Autodesk Inventor part; units mm, degrees
ref_plane "YZ Plane" through (0, 0, 0) normal (1, 0, 0) x (0, 1, 0)
ref_plane "XZ Plane" through (0, 0, 0) normal (0, 1, 0) x (-1, 0, 0)
ref_plane "XY Plane" through (0, 0, 0) normal (0, 0, 1) x (1, 0, 0)
sketch "Sketch1" plane through (0, 0, 0) normal (0, 0, 1) x (1, 0, 0)
  line L0 (0, 0) -> (50.8, 0)
  line L1 (50.8, 0) -> (50.8, 25.4)
  line L2 (50.8, 25.4) -> (0, 25.4)
  line L3 (0, 25.4) -> (0, 0)
  line L4 (3.175, 3.175) -> (47.625, 3.175)
  line L5 (47.625, 3.175) -> (47.625, 22.225)
  line L6 (47.625, 22.225) -> (3.175, 22.225)
  line L7 (3.175, 22.225) -> (3.175, 3.175)
  dimension "d0" = 50.8
  dimension "d1" = 25.4
  dimension "d2" = 3.175
  dimension "d3" = 3.175
  dimension "d4" = 3.175
  dimension "d5" = 3.175
extrude "Extrusion1" add sketch "Sketch1" along normal blind 457.2
fillet "Fillet1" radius 3.175 1 edges at (0, 25.4, 228.6)
equation "\"d3\" = d2"
equation "\"d4\" = d2"
equation "\"d5\" = d3"
properties part number "Bolt On Cross Supprot" material "Aluminum 6061"
Here's how the part is built. I have some questions about the finished solid (model axes, mm). A direction names the side the tool comes from. Round coordinates to 2 decimals unless told otherwise and drop trailing zeros. Order: outer loops, then holes, each group sorted by start corner. A loop starts at its lowest first (then second) coordinate and runs counter-clockwise, first axis right, second up. Notation, with made-up numbers: (-24.5, 21.5) -> (18.5, 21.5) arc R18 ccw to (18.5, 31.5) -> close; hole circle Ø5 at (31.5, 21.25). An arc over 180 degrees is marked (long way). Return JSON: item names as keys, results as strings.
Q1. If we mould it in two halves opening along X, with no side actions, what happens to faces 1 (the flat face through (50.8, 13, 225)), 2 (the flat face through (23, 2, 0)), 3 (the flat face through (3.175, 13, 225))? For each: released by +X, released by -X, zero draft, split by the parting line, or undercut.
Filled sheet:
{"face 1": "released by +X", "face 2": "zero draft", "face 3": "undercut"}
Q2. If we section it at A-A on y = 16.75: List the corners of the cut face in (x, z) for me (3 decimals).
Filled sheet:
{"outline": "(0, 0) -> (3.175, 0) -> (3.175, 457.2) -> (0, 457.2) -> close; (47.625, 0) -> (50.8, 0) -> (50.8, 457.2) -> (47.625, 457.2) -> close"}
Q3. I need wall thicknesses on line 1 along X through (y, z) = (5.75, 178.5) (3 decimals); line 2 along Y through (x, z) = (20.5, 285) (3 decimals). Which ranges of each line are inside material? Lowest first, please. Write a range as from..to.
Filled sheet:
{"line 1": "x = 0..3.175, 47.625..50.8", "line 2": "y = 0..3.175, 22.225..25.4"}
Q4. For pin 1 Ø6 at (y, z) = (18.5, 330) entering from -X, with a flat end and sliding along its axis, tell me the tip position at first contact or that it passes through.
Filled sheet:
{"pin 1": "stops at x = 0"}
Q5. If we section it at B-B on z = 418: List the corners of the cut face in (x, y) for me (3 decimals).
Filled sheet:
{"outline": "(0, 0) -> (50.8, 0) -> (50.8, 25.4) -> (3.175, 25.4) arc R3.175 ccw to (0, 22.225) -> close; hole (3.175, 3.175) -> (47.625, 3.175) -> (47.625, 22.225) -> (3.175, 22.225) -> close"}
Q6. If we section it at C-C on x = 31.5: List the corners of the cut face in (y, z) for me (3 decimals), plus the area to 3 significant figures.
Filled sheet:
{"outline": "(0, 0) -> (3.175, 0) -> (3.175, 457.2) -> (0, 457.2) -> close; (22.225, 0) -> (25.4, 0) -> (25.4, 457.2) -> (22.225, 457.2) -> close", "area": "2,900 mm^2"}
Q7. Which directions (+Z, -Z, +X, -X, +Y, -Y) give clear straight access to the entire face, cutting with the end or side of a thin tool? Please do faces 4 (the flat face through (25, 0, 225)), 5 (the flat face through (47.625, 13, 225)).
Filled sheet:
{"face 4": "+Z, -Z, +X, -X, -Y", "face 5": "+Z, -Z"}
